Verification items for the finished model (mm, model axes). Round coordinates to 2 decimals unless told otherwise and drop trailing zeros. Order: outer loops, then holes, each group sorted by start corner. A loop starts at its lowest first (then second) coordinate and runs counter-clockwise, first axis right, second up. Notation, with made-up numbers: M 22.5,25.25 L 71.5,25.25 A21 cw 71.5,37.25 Z; hole C 19,-17.75 d11. An arc over 180 degrees is marked long. Answer as a JSON object with one key per item and string values. Group by question number.
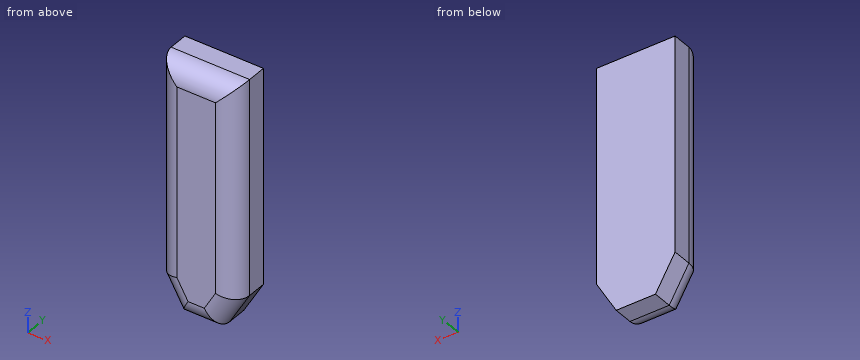
```python
from build123d import *

# Parameters (mm, degrees)
BOSS_EXTRUDE1_DEPTH = 10
FILLET1_R           = 5.08


with BuildPart() as part:
    # Sketch1 → Boss-Extrude1 (new body)
    with BuildSketch(Plane(origin=(0, 0, 0), x_dir=(1, 0, 0), z_dir=(0, 1, 0))):
        Polygon((10, -27.419872981), (10, 27.419872981), (5, 36.080127019), (-5, 36.080127019), (-10, 27.419872981), (-10, -27.419872981), align=None)
    extrude(amount=BOSS_EXTRUDE1_DEPTH)

    # Fillet1
    fillet1_edges = [part.edges().sort_by_distance(p)[0] for p in [
        (-10, 0, 0),
        (-7.5, 0, -31.75),
        (0, 0, -36.080127019),
        (7.5, 0, -31.75),
        (10, 0, 0),
        (0, 0, 27.419872981),
    ]]
    fillet(fillet1_edges, radius=FILLET1_R)


solid = part.part
```
Q1. Cross-section at B-B, the plane y = 6.25. Record the cut outline in (x, z), then the cut area to 3 significant figures.
Q2. Thickness scan on line 1 (Y direction, x = 3.5, z = -32); line 2 (Z direction, x = 3, y = 2); line 3 (X direction, y = 4.25, z = 2.5). Record the ranges inside material, lowest first. Write a range as from..to.
Q3. Cross-section at A-A, the plane x = 1.25. Record the cut outline in (y, z).
Q4. Gauge pin test, flat ends, axial feed: pin 1 Ø10 at (x, z) = (-7, 0) entering from -Y; pin 2 Ø1 at (y, z) = (1, 14) entering from +X; pin 3 Ø4 at (y, z) = (1, -11.5) entering from -X; pin 4 Ø1 at (y, z) = (5.5, -29.5) entering from -X. Record the tip position at first contact, or that the pin passes through.
Conclusion:
{
 "1": {"outline": "M -10,-27.42 L -5,-36.08 L 5,-36.08 L 10,-27.42 L 10,27.42 L -10,27.42 Z", "area": "1,230 mm2"},
 "2": {"line 1": "0.31..10", "line 2": "-35.04..26.38", "line 3": "-9.93..9.93"},
 "3": {"outline": "M 0,-31 A5.08 ccw 5.08,-36.08 L 10,-36.08 L 10,27.42 L 5.08,27.42 A5.08 ccw 0,22.34 Z"},
 "4": {"pin 1": "y = 0", "pin 2": "x = 8.52", "pin 3": "x = -9.55", "pin 4": "x = -9.09"}
}
